Work out the finished part from the listing and answer in its coordinate system (mm). A direction names the side the tool comes from. Coordinates: 2 decimals unless noted, no trailing zeros. Loops run counter-clockwise (first coordinate to the right, second up) from the corner with the lowest first, then second, coordinate; pieces in that order, holes last. Notation, with made-up numbers: (36, -39) -> (69, -39) arc R14 ccw to (69, -16) -> close; hole circle Ø3 at (-4.75, 44). An arc over 180 degrees is marked (long way). One line per question, with ' | ' between items.
```python
from build123d import *

# Parameters (mm, degrees)
SKETCH5_W            = 82
SKETCH5_H            = 23.8
BOSS_EXTRUDE1_DEPTH  = 3.9
M2_TAPPED_HOLE1_D    = 1.6
LPATTERN1_COUNT      = 2
LPATTERN1_PITCH      = 8
LPATTERN1_COUNT_DIR2 = 2
LPATTERN1_PITCH_DIR2 = 8
CUT_EXTRUDE2_START   = 3.9
REF_JOIN_CUT_FRONT_W = 18.4
REF_JOIN_CUT_FRONT_H = 18.3
CUT_EXTRUDE2_DEPTH   = 1.95
M3_TAPPED_HOLE2_D    = 2.5
LPATTERN2_COUNT      = 2
LPATTERN2_PITCH      = 8
CUT_EXTRUDE4_DEPTH   = 100.788877136
FILLET4_R            = 1
FILLET6_R            = 1


with BuildPart() as part:
    # Sketch5 → Boss-Extrude1 (new body)
    with BuildSketch(Plane(origin=(0, 0, 0), x_dir=(1, 0, 0), z_dir=(0, 1, 0))):
        with Locations((-58, 0)):
            Rectangle(SKETCH5_W, SKETCH5_H)
    extrude(amount=BOSS_EXTRUDE1_DEPTH)

    # M2 Tapped Hole1 (through all)
    with Locations(Plane(origin=(0, 3.9, 0), x_dir=(1, 0, 0), z_dir=(0, 1, 0))):
        with Locations((-20, 4)):
            m2_tapped_hole1 = Hole(M2_TAPPED_HOLE1_D / 2)

    # LPattern1: M2 Tapped Hole1 2 × 2
    with Locations(*[(-j * LPATTERN1_PITCH_DIR2, 0, i * LPATTERN1_PITCH) for i in range(LPATTERN1_COUNT) for j in range(LPATTERN1_COUNT_DIR2) if (i, j) != (0, 0)]):
        add(m2_tapped_hole1, mode=Mode.SUBTRACT)

    # Ref join cut, Front → Cut-Extrude2 (cut)
    with BuildSketch(Plane(origin=(0, 0, 0), x_dir=(-1, 0, 0), z_dir=(0, 1, 0)).offset(CUT_EXTRUDE2_START)):
        with Locations((26.2, 0)):
            Rectangle(REF_JOIN_CUT_FRONT_W, REF_JOIN_CUT_FRONT_H)
    extrude(amount=-CUT_EXTRUDE2_DEPTH, mode=Mode.SUBTRACT)

    # M3 Tapped Hole2 (through all)
    with Locations(Plane(origin=(0, 3.9, 0), x_dir=(1, 0, 0), z_dir=(0, 1, 0))):
        with Locations((-90, 4)):
            m3_tapped_hole2 = Hole(M3_TAPPED_HOLE2_D / 2)

    # LPattern2: M3 Tapped Hole2 ×2
    with Locations(*[(0, 0, i * LPATTERN2_PITCH) for i in range(1, LPATTERN2_COUNT)]):
        add(m3_tapped_hole2, mode=Mode.SUBTRACT)

    # Sketch13 → Cut-Extrude4 (cut, through all)
    with BuildSketch(Plane(origin=(0, 3.9, 0), x_dir=(1, 0, 0), z_dir=(0, 1, 0))):
        Polygon((-88, -11.9), (-88, -7.9), (-95, -7.9), (-95, 7.9), (-88, 7.9), (-88, 11.9), (-99, 11.9), (-99, -11.9), align=None)
    extrude(amount=-CUT_EXTRUDE4_DEPTH, mode=Mode.SUBTRACT)

    # Fillet4
    fillet4_edges = [part.edges().sort_by_distance(p)[0] for p in [
        (-88, 1.95, 11.9),
        (-88, 1.95, -11.9),
        (-88, 1.95, -7.9),
        (-95, 1.95, -7.9),
        (-95, 1.95, 7.9),
        (-88, 1.95, 7.9),
    ]]
    fillet(fillet4_edges, radius=FILLET4_R)

    # Fillet6
    fillet6_edges = [part.edges().sort_by_distance(p)[0] for p in [
        (-35.4, 2.925, -9.15),
        (-17, 2.925, -9.15),
        (-17, 2.925, 9.15),
        (-35.4, 2.925, 9.15),
        (-17, 1.95, -11.9),
        (-17, 1.95, 11.9),
    ]]
    fillet(fillet6_edges, radius=FILLET6_R)


solid = part.part
```
1) For faces 1 (the face through (-26, 1.95, -2)), 2 (the face through (-88, 2, -10)), 3 (the face through (-91.155, 1.923, 4.479)), 4 (the face through (-88, 2, 10)), 5 (the face through (-53, 2, -11.9)), determine the directions among +Z, -Z, +X, -X, +Y, -Y from which every point of the face is accessible in a straight line to the end or side of a thin tool.
Check values:
face 1: +X, +Y | face 2: -Z, -X, +Y, -Y | face 3: +Y, -Y | face 4: +Z, -X, +Y, -Y | face 5: -Z, +X, -X, +Y, -Y
2) Find section A-A (x = -20). Write down the section's boundary in (y, z).
Check values:
outline: (0, -11.9) -> (3.9, -11.9) -> (3.9, -9.15) -> (1.95, -9.15) -> (1.95, -4.8) -> (0, -4.8) -> close; (0, -3.2) -> (1.95, -3.2) -> (1.95, 3.2) -> (0, 3.2) -> close; (0, 4.8) -> (1.95, 4.8) -> (1.95, 9.15) -> (3.9, 9.15) -> (3.9, 11.9) -> (0, 11.9) -> close
3) The mould has two halves that part along Z. Classify faces 6 (the face through (-53, 2, 11.9)), 7 (the face through (-35.4, 3, 0)), 8 (the face through (-95, 2, 0)): released by +Z, released by -Z, zero draft, split by the parting line, or undercut.
Check values:
face 6: released by +Z | face 7: undercut | face 8: zero draft
4) Find section D-D (x = -90). Write down the section's boundary in (y, z).
Check values:
outline: (0, -7.9) -> (3.9, -7.9) -> (3.9, -5.25) -> (0, -5.25) -> close; (0, -2.75) -> (3.9, -2.75) -> (3.9, 2.75) -> (0, 2.75) -> close; (0, 5.25) -> (3.9, 5.25) -> (3.9, 7.9) -> (0, 7.9) -> close
5) Find section C-C (y = 0.7). Write down the section's boundary in (x, z), plus the area to 3 significant figures.
Check values:
outline: (-95, -6.9) arc R1 ccw to (-94, -7.9) -> (-89, -7.9) arc R1 cw to (-88, -8.9) -> (-88, -10.9) arc R1 ccw to (-87, -11.9) -> (-18, -11.9) arc R1 ccw to (-17, -10.9) -> (-17, 10.9) arc R1 ccw to (-18, 11.9) -> (-87, 11.9) arc R1 ccw to (-88, 10.9) -> (-88, 8.9) arc R1 cw to (-89, 7.9) -> (-94, 7.9) arc R1 ccw to (-95, 6.9) -> close; hole circle Ø2.5 at (-90, -4); hole circle Ø2.5 at (-90, 4); hole circle Ø1.6 at (-28, -4); hole circle Ø1.6 at (-28, 4); hole circle Ø1.6 at (-20, -4); hole circle Ø1.6 at (-20, 4) | area: 1,780 mm^2
6) Flat-ended cylindrical pins translate along their axes: pin 1 (2 mm diameter, centred on y = 3, z = 4, fed in from +X); pin 2 (9 mm diameter, centred on x = -24.5, z = 3, fed in from +Y); pin 3 (0.6 mm diameter, centred on y = 1.5, z = 10.5, fed in from -X). Find the tip coordinate at first contact, or state that the pin passes through.
Check values:
pin 1: stops at x = -35.4 | pin 2: stops at y = 1.95 | pin 3: stops at x = -88
7) Find section B-B (z = 4). Write down the section's boundary in (x, y), plus the area to 3 significant figures.
Check values:
outline: (-95, 0) -> (-91.25, 0) -> (-91.25, 3.9) -> (-95, 3.9) -> close; (-88.75, 0) -> (-28.8, 0) -> (-28.8, 1.95) -> (-35.4, 1.95) -> (-35.4, 3.9) -> (-88.75, 3.9) -> close; (-27.2, 0) -> (-20.8, 0) -> (-20.8, 1.95) -> (-27.2, 1.95) -> close; (-19.2, 0) -> (-17, 0) -> (-17, 1.95) -> (-19.2, 1.95) -> close | area: 252 mm^2
8) Find the intervals of material crossed by line 1 along Z through (x, y) = (-90, 2.4); line 2 along Z through (x, y) = (-28, 1.3); line 3 along X through (y, z) = (1.1, 4), in increasing order.
Check values:
line 1: z = -7.9 to -5.25, -2.75 to 2.75, 5.25 to 7.9 | line 2: z = -11.9 to -4.8, -3.2 to 3.2, 4.8 to 11.9 | line 3: x = -95 to -91.25, -88.75 to -28.8, -27.2 to -20.8, -19.2 to -17
